The listing builds one solid part. Answer for the finished solid, in the listing's coordinates (mm). A direction names the side the tool comes from. Give positions to 0.01 mm unless a question says otherwise; leave off trailing zeros. Order: outer loops, then holes, each group sorted by start corner. A loop starts at its lowest first (then second) coordinate and runs counter-clockwise, first axis right, second up.
```python
from build123d import *

# Parameters (mm, degrees)
F0_W     = 76.2
F0_H     = 76.2
F1_DEPTH = 76.2
F2_W     = 25.4
F2_H     = 25.4
F3_DEPTH = 12.7
F4_R     = 12.7
F5_DEPTH = 12.7


with BuildPart() as f1:
    # F0 (on Front) → F1 (new body)
    with BuildSketch(Plane.XZ):
        with Locations((-38.1, 39.819894)):
            Rectangle(F0_W, F0_H)
    extrude(amount=F1_DEPTH)

    # F2 (on face) → F3 (join)
    with BuildSketch(Plane.XZ.offset(76.2)):
        with Locations((-38.1, 39.819894)):
            Rectangle(F2_W, F2_H)
    extrude(amount=F3_DEPTH)

    # F4 (on face) → F5 (join)
    with BuildSketch(Plane.YZ):
        with Locations((-38.1, 39.819894)):
            Circle(F4_R)
    extrude(amount=F5_DEPTH)


solid = f1.part
```
1) Straight lines are drawn through the part: probe 1 along Y at (x, z) = (-58.5, 61.5); probe 2 along Z at (x, y) = (-31, -83.5). For each, find the intervals that lie inside material, in ascending order.
Geometry says:
probe 1: y = -76.2 to 0
probe 2: z = 27.12 to 52.52
2) Given P1, Ø10, axis at y = -80.5, z = 38.5, coming from the +X side; P2, Ø6.5, axis at x = -39, y = -79.5, coming from the -Z side; P3, Ø2, axis at x = -56, z = 11, coming from the -Y side, each flat-ended and moving along its own axis, determine where each tip first touches the part or whether it passes through.
Geometry says:
P1: stops at x = 0
P2: stops at z = 27.12
P3: stops at y = -76.2
3) Find section D-D (z = 47). Write down the section's boundary in (x, y), then the cut area to 3 significant figures.
Geometry says:
outline: (-76.2, -76.2) - (-50.8, -76.2) - (-50.8, -88.9) - (-25.4, -88.9) - (-25.4, -76.2) - (0, -76.2) - (0, -48.58) - (12.7, -48.58) - (12.7, -27.62) - (0, -27.62) - (0, 0) - (-76.2, 0) - close
area: 6,400 mm2
4) Find section B-B (y = -38.1). Write down the section's boundary in (x, z).
Geometry says:
outline: (-76.2, 1.72) - (0, 1.72) - (0, 27.12) - (12.7, 27.12) - (12.7, 52.52) - (0, 52.52) - (0, 77.92) - (-76.2, 77.92) - close
5) Find section A-A (z = 33.5). Write down the section's boundary in (x, y), then the cut area to 3 significant figures.
Geometry says:
outline: (-76.2, -76.2) - (-50.8, -76.2) - (-50.8, -88.9) - (-25.4, -88.9) - (-25.4, -76.2) - (0, -76.2) - (0, -49.12) - (12.7, -49.12) - (12.7, -27.08) - (0, -27.08) - (0, 0) - (-76.2, 0) - close
area: 6,410 mm2
6) A tool of negligible diameter and unlimited length cuts with its end or side. For faces 1 (the flat face through (-38, -82, 27.12)), 2 (the flat face through (0, -38, 22)), 3 (the flat face through (-38, -82, 52.52)), 4 (the flat face through (-25.4, -82, 40)), from which of +Z, -Z, +X, -X, +Y, -Y can it reach the whole face along a straight path? Write none if from no direction.
Geometry says:
face 1: -Z, +X, -X, -Y
face 2: +X
face 3: +Z, +X, -X, -Y
face 4: +Z, -Z, +X, -Y
7) Find section C-C (x = -38). Write down the section's boundary in (y, z).
Geometry says:
outline: (-88.9, 27.12) - (-76.2, 27.12) - (-76.2, 1.72) - (0, 1.72) - (0, 77.92) - (-76.2, 77.92) - (-76.2, 52.52) - (-88.9, 52.52) - close
